from build123d import *

# Parameters (mm, degrees)
BOSS_EXTRUDE1_DEPTH = 1


with BuildPart() as part:
    # Sketch1 → Boss-Extrude1 (new body)
    with BuildSketch(Plane.XY):
        with BuildLine():
            Line((0, 11.8375), (0, 17.5))
            Line((0, 17.5), (20, 17.5))
            Line((20, 17.5), (20, 0))
            Line((20, 0), (0, 0))
            Line((0, 0), (0, 5.6625))
            ThreePointArc((0, 5.6625), (-0.464967985, 6.785032015), (-1.5875, 7.25))
            Line((-1.5875, 7.25), (-10, 7.25))
            Line((-10, 7.25), (-10, 10.25))
            Line((-10, 10.25), (-1.5875, 10.25))
            ThreePointArc((-1.5875, 10.25), (-0.464967985, 10.714967985), (0, 11.8375))
        make_face()
    extrude(amount=BOSS_EXTRUDE1_DEPTH)


solid = part.part
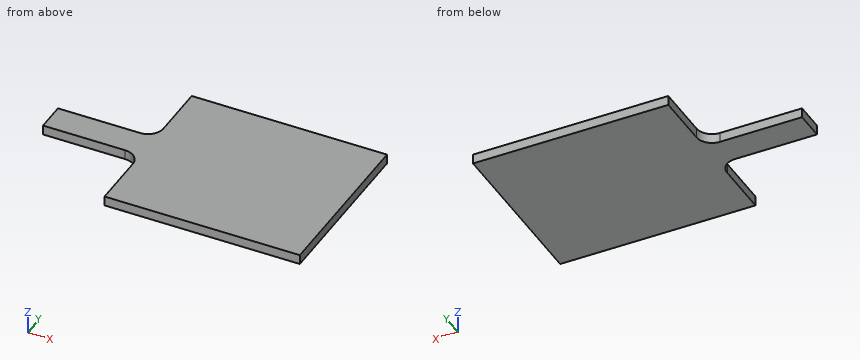
CAD build for the part. Positions are in the model's coordinates, mm. Give positions to 0.01 mm unless a question says otherwise; leave off trailing zeros. Order: outer loops, then holes, each group sorted by start corner. A loop starts at its lowest first (then second) coordinate and runs counter-clockwise, first axis right, second up. Notation, with made-up numbers: (86.5, 0.25) -> (142.5, 0.25) arc R28 ccw to (142.5, 22.25) -> close; hole circle Ø1 at (-20, -17.75). An arc over 180 degrees is marked (long way). Return JSON: item names as keys, results as strings.
Q1. Drill centre lines: line 1 (Y direction, x = -8, z = 0.55); line 2 (X direction, y = 1.75, z = 0.1); line 3 (X direction, y = 6.75, z = 0.5). Where is each one in solid material? Low to high.
Working result:
{"line 1": "7.25 to 10.25", "line 2": "0 to 20", "line 3": "-0.43 to 20"}
Q2. Flat gauge pins, fed straight in: pin 1 (0.5 mm diameter, centred on x = -6, z = 0.5, fed in from -Y); pin 2 (0.5 mm diameter, centred on x = -5, z = 0.5, fed in from +Y). Where does each tip first touch, or does it go through?
Working result:
{"pin 1": "y = 7.25", "pin 2": "y = 10.25"}
Q3. Saw through at B-B (x = -4.25). Write the cut outline in (y, z).
Working result:
{"outline": "(7.25, 0) -> (10.25, 0) -> (10.25, 1) -> (7.25, 1) -> close"}
Q4. Saw through at C-C (y = 3). Write the cut outline in (x, z).
Working result:
{"outline": "(0, 0) -> (20, 0) -> (20, 1) -> (0, 1) -> close"}
